```python
from build123d import *

# Parameters (mm, degrees)
F0_W     = 25.4
F0_H     = 25.4
F1_DEPTH = 6.35
F2_R     = 3.302
F3_DEPTH = 25.4
F4_W     = 3.175
F4_H     = 12.7
F5_DEPTH = 12.7
F6_W     = 4.7625
F6_H     = 3.175
F7_DEPTH = 6.604


with BuildPart() as f1:
    # F0 (on Right) → F1 (new body)
    with BuildSketch(Plane.YZ):
        with Locations((5.450736, 3.029342)):
            Rectangle(F0_W, F0_H)
    extrude(amount=F1_DEPTH)

    # F2 (on face) → F3 (cut)
    with BuildSketch(Plane.YZ.offset(6.35)):
        with Locations((-0.645264, 9.125342)):
            Circle(F2_R)
    extrude(amount=-F3_DEPTH, mode=Mode.SUBTRACT)

    # F4 (on face) → F5 (cut)
    with BuildSketch(Plane.XY.offset(15.729342)):
        with Locations((3.175, -0.899264)):
            Rectangle(F4_W, F4_H)
    extrude(amount=-F5_DEPTH, mode=Mode.SUBTRACT)

    # F6 (on face) → F7 (cut)
    with BuildSketch(Plane.XY.offset(15.729342)):
        with Locations((3.96875, -0.645264)):
            Rectangle(F6_W, F6_H)
    extrude(amount=-F7_DEPTH, mode=Mode.SUBTRACT)


solid = f1.part
```
CAD build for the part. Positions are in the model's coordinates, mm. A direction names the side the tool comes from. Round coordinates to 2 decimals unless told otherwise and drop trailing zeros. Loops run counter-clockwise (first coordinate to the right, second up) from the corner with the lowest first, then second, coordinate; pieces in that order, holes last. Notation, with made-up numbers: (13.5, 48) - (39.5, 48) arc R4 ccw to (39.5, 53) - close; hole circle Ø4 at (-13, -29). An arc over 180 degrees is marked (long way). Return JSON: item names as keys, results as strings. Group by question number.
Q1. Band-saw the part on A-A on z = 3.5. Give the cut face in (x, y).
Q2. Tool access for faces 1 (the face through (3, -1, 3.029)), 2 (the face through (5.567, -0.767, 5.826)), 3 (the face through (6, -2.233, 14)): list every direction of +Z, -Z, +X, -X, +Y, -Y with a clear straight run to the whole face (end or side of a thin tool).
Q3. Two-plate mould, pull along X, no slides. Class faces 4 (the face through (6, 0.942, 14)), 5 (the face through (3, 5.451, 9)), 6 (the face through (0, 5, 3)): +X half, -X half, draft (parallel to the pull), parting line (faces both ways), or undercut.
Q4. Band-saw the part on C-C on x = 3.75. Give the cut face in (y, z), plus the area to 3 significant figures.
Q5. Band-saw the part on D-D on y = -4.5. Give the cut face in (x, z), plus the area to 3 significant figures.
Q6. Drill centre lines: line 1 along Y through (x, z) = (5.75, 13); line 2 along X through (y, z) = (3.75, 7.25); line 3 along Y through (x, z) = (4, 5.75). Where is each one in solid material? Low to high. Write a range as [from, to].
Q7. Band-saw the part on B-B on y = 0. Give the cut face in (x, z), plus the area to 3 significant figures.
Solutions:
{
 "1": {"outline": "(0, -7.25) - (1.59, -7.25) - (1.59, 5.45) - (4.76, 5.45) - (4.76, -7.25) - (6.35, -7.25) - (6.35, 18.15) - (0, 18.15) - close"},
 "2": {"face 1": "+Z, -Y", "face 2": "+X, -X", "face 3": "+Z, +X"},
 "3": {"face 4": "draft", "face 5": "undercut", "face 6": "-X half"},
 "4": {"outline": "(-7.25, -9.67) - (18.15, -9.67) - (18.15, 15.73) - (5.45, 15.73) - (5.45, 3.03) - (-7.25, 3.03) - close", "area": "484 mm^2"},
 "5": {"outline": "(0, -9.67) - (6.35, -9.67) - (6.35, 15.73) - (4.76, 15.73) - (4.76, 3.03) - (1.59, 3.03) - (1.59, 15.73) - (0, 15.73) - close", "area": "121 mm^2"},
 "6": {"line 1": "y = [-7.25, -2.23], [0.94, 18.15]", "line 2": "x = [0, 1.59], [4.76, 6.35]", "line 3": "y = [5.45, 18.15]"},
 "7": {"outline": "(0, -9.67) - (6.35, -9.67) - (6.35, 5.89) - (4.76, 5.89) - (4.76, 3.03) - (1.59, 3.03) - (1.59, 5.89) - (0, 5.89) - close; (0, 12.36) - (1.59, 12.36) - (1.59, 15.73) - (0, 15.73) - close", "area": "95.1 mm^2"}
}
